Study the drawing (mm; zero at the part's minimum x, y, z) and answer. Round coordinates to 2 decimals unless told otherwise and drop trailing zeros. Order: outer loops, then holes, each group sorted by start corner. A loop starts at its lowest first (then second) coordinate and runs counter-clockwise, first axis right, second up. Notation, with made-up numbers: (79.25, 89.25) -> (100.25, 89.25) arc R7 cw to (100.25, 96.25) -> close; hole circle Ø11 at (-7, -6). An arc over 180 degrees is marked (long way). Answer in a Markdown table with one row per item. Add a question column.
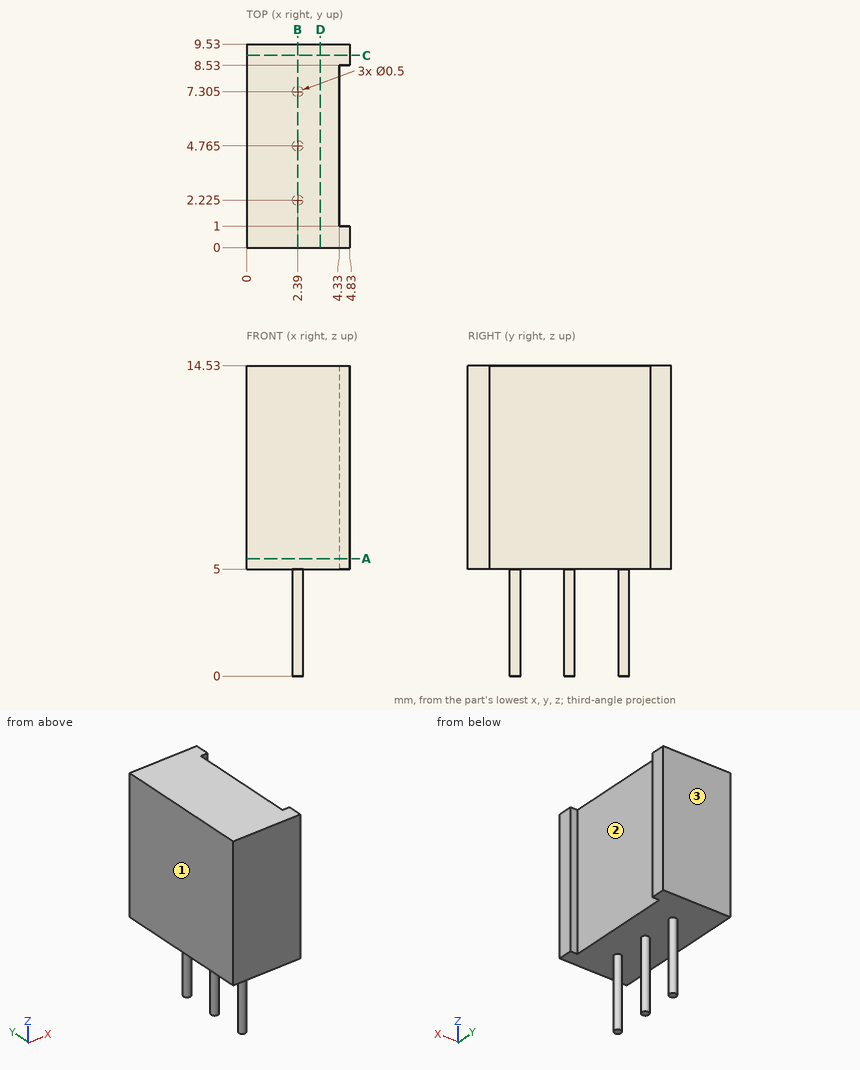
Item 1: The part is cut by section C-C, the plane y = 9. Give the vertices of the cut face in (x, z), and give its area (3 significant figures).
Item 2: The part is cut by section D-D, the plane x = 3.45. Give the vertices of the cut face in (y, z).
Item 3: The part is cut by section B-B, the plane x = 2.39. Give the vertices of the cut face in (y, z) (3 decimals), and give its area (3 significant figures).
Item 4: Find the intervals of material crossed by probe 1 along Z at (x, y) = (3.65, 6.5); probe 2 along X at (y, z) = (8.25, 10.75), in increasing order. Write a range as [from, to].
Item 5: For a pull along Y with two mould halves and no side action, classify the marked faces 1, 2 and 3 as released by +Y, released by -Y, zero draft, split by the parting line, or undercut.
Item 6: Flat-ended cylindrical pins translate along their axes: P1, Ø2.5, axis at y = 4.5, z = 10, coming from the +X side; P2, Ø2, axis at x = 3.5, z = 3, coming from the +Y side; P3, Ø1.4, axis at x = 1.5, y = 6.5, coming from the -Z side. Find the tip coordinate at first contact, or state that the pin passes through.
Item 7: The part is cut by section A-A, the plane z = 5.5. Give the vertices of the cut face in (x, y), and give its area (3 significant figures).
Resolved:
| question | item | result |
|---|---|---|
| 1 | outline | (0, 5) -> (4.83, 5) -> (4.83, 14.53) -> (0, 14.53) -> close |
| 1 | area | 46.0 mm2 |
| 2 | outline | (0, 5) -> (9.53, 5) -> (9.53, 14.53) -> (0, 14.53) -> close |
| 3 | outline | (0, 5) -> (1.975, 5) -> (1.975, 0) -> (2.475, 0) -> (2.475, 5) -> (4.515, 5) -> (4.515, 0) -> (5.015, 0) -> (5.015, 5) -> (7.055, 5) -> (7.055, 0) -> (7.555, 0) -> (7.555, 5) -> (9.53, 5) -> (9.53, 14.53) -> (0, 14.53) -> close |
| 3 | area | 98.3 mm2 |
| 4 | probe 1 | [5, 14.53] |
| 4 | probe 2 | [0, 4.33] |
| 5 | face 1 | zero draft |
| 5 | face 2 | undercut |
| 5 | face 3 | released by +Y |
| 6 | P1 | x = 4.33 |
| 6 | P2 | y = 7.53 |
| 6 | P3 | z = 5 |
| 7 | outline | (0, 0) -> (4.83, 0) -> (4.83, 1) -> (4.33, 1) -> (4.33, 8.53) -> (4.83, 8.53) -> (4.83, 9.53) -> (0, 9.53) -> close |
| 7 | area | 42.3 mm2 |
